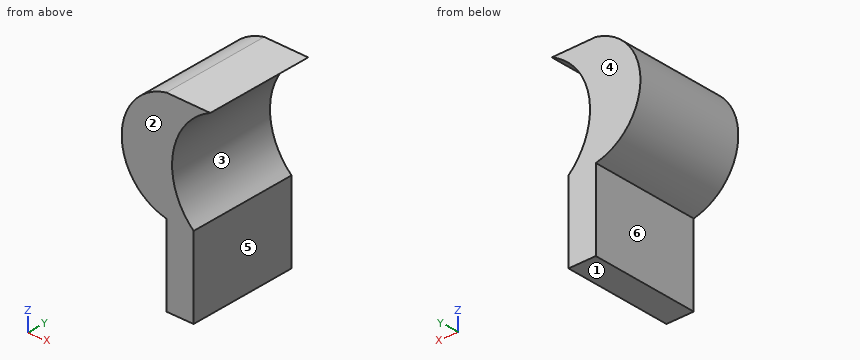
```python
from build123d import *

# Parameters (mm, degrees)
F1_DEPTH = 76.2


with BuildPart() as f1:
    # F0 (on Front) → F1 (new body)
    with BuildSketch(Plane.XZ):
        with BuildLine():
            Line((-29.08165, -56.035373), (-29.08165, 0))
            ThreePointArc((-29.08165, 0), (-43.520037, 40.922253), (-17.44899, 75.612284))
            Line((-17.44899, 75.612284), (-48.091117, 75.89601))
            ThreePointArc((-48.091117, 75.89601), (-79.137953, 37.948005), (-48.091117, 0))
            Line((-48.091117, 0), (-48.091117, -56.035373))
            Line((-48.091117, -56.035373), (-29.08165, -56.035373))
        make_face()
    extrude(amount=F1_DEPTH)


solid = f1.part
```
The listing builds one solid part. Answer for the finished solid, in the listing's coordinates (mm). Face numbers are marked on the shaded views. A direction names the side the tool comes from. Coordinates: 2 decimals unless noted, no trailing zeros. Loops run counter-clockwise (first coordinate to the right, second up) from the corner with the lowest first, then second, coordinate; pieces in that order, holes last. Notation, with made-up numbers: (-11.75, 78) - (19.25, 78) arc R32 cw to (19.25, 110) - close; hole circle Ø11 at (89.25, 46.5). An arc over 180 degrees is marked (long way). Use a Markdown table: item, result. Add a question column.
1) The mould has two halves that part along Z. Classify the marked faces 1, 2 and 3: released by +Z, released by -Z, zero draft, split by the parting line, or undercut.
2) Given pin 1 (1 mm diameter, centred on x = -33.5, y = -26.5, fed in from +Z); pin 2 (5 mm diameter, centred on y = -45.5, z = -1.5, fed in from +X); pin 3 (2 mm diameter, centred on x = -42.5, z = 49, fed in from +Y); pin 4 (4 mm diameter, centred on y = -27, z = 41.5, fed in from +X), each flat-ended and moving along its own axis, determine where each tip first touches the part or whether it passes through.
3) The part is cut by section A-A, the plane x = -32. Give the vertices of the cut face in (y, z).
4) Find the intervals of material crossed by line 1 (X direction, y = -57, z = -13); line 2 (Z direction, x = -55.5, y = -60.5); line 3 (X direction, y = -11.5, z = 28), in increasing order.
5) The part is cut by section B-B, the plane y = -16.5. Give the vertices of the cut face in (x, z) (3 decimals).
6) The part is cut by section D-D, the plane x = -24. Give the vertices of the cut face in (y, z).
7) For the marked faces 4, 5 and 6, determine the directions among +Z, -Z, +X, -X, +Y, -Y from which every point of the face is accessible in a straight line to the end or side of a thin tool.
8) The part is cut by section C-C, the plane z = -34. Give the vertices of the cut face in (x, y), and give its area (3 significant figures).
Here are the results:
| question | item | result |
|---|---|---|
| 1 | face 1 | released by -Z |
| 1 | face 2 | zero draft |
| 1 | face 3 | undercut |
| 2 | pin 1 | stops at z = 75.77 |
| 2 | pin 2 | stops at x = -29.08 |
| 2 | pin 3 | stops at y = 0 |
| 2 | pin 4 | stops at x = -43.05 |
| 3 | outline | (-76.2, -56.04) - (0, -56.04) - (0, 2.91) - (-76.2, 2.91) - close; (-76.2, 64.96) - (0, 64.96) - (0, 75.75) - (-76.2, 75.75) - close |
| 4 | line 1 | x = -48.09 to -29.08 |
| 4 | line 2 | z = 2.29 to 73.61 |
| 4 | line 3 | x = -77.84 to -43.67 |
| 5 | outline | (-48.091, -56.035) - (-29.082, -56.035) - (-29.082, 0) arc R45.945 cw to (-17.449, 75.612) - (-48.091, 75.896) arc R38.715 ccw to (-48.091, 0) - close |
| 6 | outline | (-76.2, 71.89) - (0, 71.89) - (0, 75.67) - (-76.2, 75.67) - close |
| 7 | face 4 | +Z, -Z, +X, -X, +Y |
| 7 | face 5 | -Z, +X, +Y, -Y |
| 7 | face 6 | -Z, -X, +Y, -Y |
| 8 | outline | (-48.09, -76.2) - (-29.08, -76.2) - (-29.08, 0) - (-48.09, 0) - close |
| 8 | area | 1,450 mm^2 |
